Here's how the part is built. I have some questions about the finished solid (model axes, mm). A direction names the side the tool comes from. Coordinates: 2 decimals unless noted, no trailing zeros. Order: outer loops, then holes, each group sorted by start corner. A loop starts at its lowest first (then second) coordinate and runs counter-clockwise, first axis right, second up. Notation, with made-up numbers: (-3.75, 50.5) - (38.25, 50.5) arc R11 cw to (38.25, 61.5) - close; hole circle Ø3 at (17.25, 49.25). An arc over 180 degrees is marked (long way). Answer as CSV lines item,"result". Start each with the question number.
Q1. Thinking about a two-plate mould opening in X: for faces 3 (the face through (-25, 0, 2)), 4 (the face through (-2.213, 12.88, 1.61)), 5 (the face through (0, 11, 0)), which applies, released by +X, released by -X, zero draft, split by the parting line, or undercut?
Q2. Suppose I cut it at A-A (y = 20). Please give me the cut outline in (x, z) (3 decimals), then the cut area to 3 significant figures.
Q3. For pin 1 Ø15.5 at (x, y) = (0, 0) entering from +Z, with a flat end and sliding along its axis, tell me the tip position at first contact or that it passes through.
Q4. For faces 1 (the face through (0, -25, 2)), 2 (the face through (-13.585, -5.484, 1.61)), which set-ups out of +Z, -Z, +X, -X, +Y, -Y let a thin tool reach every point of the face, with its end or its side?
Q5. I need wall thicknesses on line 1 (Y direction, x = -20, z = 0.8); line 2 (Y direction, x = -7, z = 1.35); line 3 (X direction, y = -22, z = 2.7). Which ranges of each line are inside material? Lowest first, please.
Q6. Suppose I cut it at C-C (z = 2.1). Count the separate pieces of the cut face and the enclosed holes in it, then the cut area to 3 significant figures.
Q7. Suppose I cut it at B-B (x = 0). Please give me the cut outline in (y, z) (3 decimals).
from build123d import *

# Parameters (mm, degrees)
SKETCH1_W           = 50
SKETCH1_H           = 50
BOSS_EXTRUDE1_DEPTH = 3.175
SKETCH2_R           = 9.75
CUT_EXTRUDE1_DEPTH  = 36.497614356
CUT_EXTRUDE2_DEPTH  = 36.497614356
SKETCH4_R           = 2.25
CUT_EXTRUDE3_DEPTH  = 36.497614356


with BuildPart() as part:
    # Sketch1 → Boss-Extrude1 (new body)
    with BuildSketch(Plane.XY):
        Rectangle(SKETCH1_W, SKETCH1_H)
    extrude(amount=BOSS_EXTRUDE1_DEPTH)

    # Sketch2 → Cut-Extrude1 (cut, through all)
    with BuildSketch(Plane.XY.offset(3.175)):
        Circle(SKETCH2_R)
    extrude(amount=-CUT_EXTRUDE1_DEPTH, mode=Mode.SUBTRACT)

    # Sketch3 → Cut-Extrude2 (cut, through all)
    with BuildSketch(Plane.XY.offset(3.175)):
        with BuildLine():
            ThreePointArc((-4.283245474, 14.009864675), (-5.500937795, 13.57800366), (-6.675845238, 13.040536429))
            ThreePointArc((-6.675845238, 13.040536429), (-7.392687591, 10.819920064), (-5.172071225, 10.103077711))
            ThreePointArc((-5.172071225, 10.103077711), (-4.261818701, 10.519477238), (-3.318418849, 10.85405898))
            ThreePointArc((-3.318418849, 10.85405898), (-2.222929314, 12.91437514), (-4.283245474, 14.009864675))
        make_face()
        with BuildLine():
            ThreePointArc((14.009864675, 4.283245474), (13.57800366, 5.500937795), (13.040536429, 6.675845238))
            ThreePointArc((13.040536429, 6.675845238), (10.819920064, 7.392687591), (10.103077711, 5.172071225))
            ThreePointArc((10.103077711, 5.172071225), (10.519477238, 4.261818701), (10.85405898, 3.318418849))
            ThreePointArc((10.85405898, 3.318418849), (12.91437514, 2.222929314), (14.009864675, 4.283245474))
        make_face()
        with BuildLine():
            ThreePointArc((4.283245474, -14.009864675), (5.500937795, -13.57800366), (6.675845238, -13.040536429))
            ThreePointArc((6.675845238, -13.040536429), (7.392687591, -10.819920064), (5.172071225, -10.103077711))
            ThreePointArc((5.172071225, -10.103077711), (4.261818701, -10.519477238), (3.318418849, -10.85405898))
            ThreePointArc((3.318418849, -10.85405898), (2.222929314, -12.91437514), (4.283245474, -14.009864675))
        make_face()
        with BuildLine():
            ThreePointArc((-14.009864675, -4.283245474), (-13.57800366, -5.500937795), (-13.040536429, -6.675845238))
            ThreePointArc((-13.040536429, -6.675845238), (-10.819920064, -7.392687591), (-10.103077711, -5.172071225))
            ThreePointArc((-10.103077711, -5.172071225), (-10.519477238, -4.261818701), (-10.85405898, -3.318418849))
            ThreePointArc((-10.85405898, -3.318418849), (-12.91437514, -2.222929314), (-14.009864675, -4.283245474))
        make_face()
    extrude(amount=-CUT_EXTRUDE2_DEPTH, mode=Mode.SUBTRACT)

    # Sketch4 → Cut-Extrude3 (cut, through all)
    with BuildSketch(Plane.XY.offset(3.175)):
        with Locations((-20, 20)):
            Circle(SKETCH4_R)
        with Locations(Location((-20, -20, 0), (0, 0, 180))):
            Circle(SKETCH4_R)
        with Locations(Location((20, 20, 0), (0, 0, 180))):
            Circle(SKETCH4_R)
        with Locations((20, -20)):
            Circle(SKETCH4_R)
    extrude(amount=-CUT_EXTRUDE3_DEPTH, mode=Mode.SUBTRACT)


solid = part.part
Here are the results:
1,face 3,"released by -X"
1,face 4,"undercut"
1,face 5,"zero draft"
2,outline,"(-25, 0) - (-22.25, 0) - (-22.25, 3.175) - (-25, 3.175) - close; (-17.75, 0) - (17.75, 0) - (17.75, 3.175) - (-17.75, 3.175) - close; (22.25, 0) - (25, 0) - (25, 3.175) - (22.25, 3.175) - close"
2,area,"130 mm²"
3,pin 1,"passes through"
4,face 1,"+Z, -Z, +X, -X, -Y"
4,face 2,"+Z, -Z"
5,line 1,"y = -25 to -22.25, -17.75 to 17.75, 22.25 to 25"
5,line 2,"y = -25 to -6.79, 6.79 to 10.32, 12.82 to 25"
5,line 3,"x = -25 to -21.03, -18.97 to 18.97, 21.03 to 25"
6,separate pieces,"1"
6,enclosed holes,"9"
6,area,"2,070 mm²"
7,outline,"(-25, 0) - (-9.75, 0) - (-9.75, 3.175) - (-25, 3.175) - close; (9.75, 0) - (25, 0) - (25, 3.175) - (9.75, 3.175) - close"
